Autodesk Inventor part; units mm, degrees
ref_plane "YZ Plane" through (0, 0, 0) normal (1, 0, 0) x (0, 1, 0)
ref_plane "XZ Plane" through (0, 0, 0) normal (0, 1, 0) x (-1, 0, 0)
ref_plane "XY Plane" through (0, 0, 0) normal (0, 0, 1) x (1, 0, 0)
sketch "スケッチ1" plane through (0, 0, 0) normal (0, 1, 0) x (-1, 0, 0)
  line L0 (35, 0) -> (0, 0)
  line L1 (0, 0) -> (0, -40)
  line L2 (0, -40) -> (35, -40)
  line L3 (35, -40) -> (35, 0)
  line L4 (30, -5) -> (5, -5)
  line L5 (5, -5) -> (5, -35)
  line L6 (5, -35) -> (30, -35)
  line L7 (30, -35) -> (30, -5)
  circle A0 centre (30, -5) radius 0.8
  circle A1 centre (30, -35) radius 0.8
  circle A2 centre (5, -35) radius 0.8
  circle A3 centre (5, -5) radius 0.8
  dimension "d0" = 25
  dimension "d1" = 30
  dimension "d2" = 5
  dimension "d3" = 5
  dimension "d4" = 5
  dimension "d5" = 5
  dimension "d6" = 1.6
  dimension "d7" = 1.6
  dimension "d8" = 1.6
  dimension "d9" = 1.6
extrude "押し出し1" add sketch "スケッチ1" along normal blind 30 contours L3 L2 L1 L0 | L4 A0 L7 A1 L6 A2 L5 A3
equation "\"d3\" = d2"
equation "\"d4\" = d2"
equation "\"d5\" = d2"
properties part number "board"
Verification items for the finished model (mm, model axes). Coordinates: 2 decimals unless noted, no trailing zeros. Loops run counter-clockwise (first coordinate to the right, second up) from the corner with the lowest first, then second, coordinate; pieces in that order, holes last. Notation, with made-up numbers: (64.5, 35) -> (113.5, 35) arc R15 ccw to (113.5, 42) -> close; hole circle Ø6 at (20.5, -1). An arc over 180 degrees is marked (long way). Answer in a Markdown table with one row per item.
1) Draft check along Z on faces 1 (the face through (-18, 15, 0)), 2 (the face through (0, 15, -20)), 3 (the face through (-17, 15, -40)), 4 (the face through (-30.43, 14.79, -35.675)). Enter one of: released by +Z, released by -Z, zero draft, split by the parting line, or undercut.
The answers:
| item | result |
|---|---|
| face 1 | released by +Z |
| face 2 | zero draft |
| face 3 | released by -Z |
| face 4 | undercut |
2) Section check A-A (x = -30). Record the cut outline in (y, z), and give its area (3 significant figures).
The answers:
| item | result |
|---|---|
| outline | (0, -40) -> (30, -40) -> (30, -35.8) -> (0, -35.8) -> close; (0, -34.2) -> (30, -34.2) -> (30, -5.8) -> (0, -5.8) -> close; (0, -4.2) -> (30, -4.2) -> (30, 0) -> (0, 0) -> close |
| area | 1,100 mm2 |
3) Section check B-B (z = -5). Record the cut outline in (x, y).
The answers:
| item | result |
|---|---|
| outline | (-35, 0) -> (-30.8, 0) -> (-30.8, 30) -> (-35, 30) -> close; (-29.2, 0) -> (-5.8, 0) -> (-5.8, 30) -> (-29.2, 30) -> close; (-4.2, 0) -> (0, 0) -> (0, 30) -> (-4.2, 30) -> close |
4) Scan lines: line 1 along Z through (x, y) = (-5, 20); line 2 along X through (y, z) = (22.5, -35); line 3 along Z through (x, y) = (-29.5, 16.25). Record each from-to range of solid material in increasing order. Write a range as from..to.
The answers:
| item | result |
|---|---|
| line 1 | z = -40..-35.8, -34.2..-5.8, -4.2..0 |
| line 2 | x = -35..-30.8, -29.2..-5.8, -4.2..0 |
| line 3 | z = -40..-35.62, -34.38..-5.62, -4.38..0 |
